The model under review builds one solid part; all positions refer to its coordinate system, in mm. A direction names the side the tool comes from. Coordinates: 2 decimals unless noted, no trailing zeros. Loops run counter-clockwise (first coordinate to the right, second up) from the corner with the lowest first, then second, coordinate; pieces in that order, holes last. Notation, with made-up numbers: M 75,46 L 98,46 A27 ccw 98,72 Z; hole C 46.25,21.25 d1. An arc over 180 degrees is marked long. Use CSV: the item, a comma, the result in double quotes. Start each with the question number.
1. Draft analysis for pull direction X (two halves, no side actions). For faces 5 (the flat face through (-32, 2, -32.258)), 6 (the flat face through (-42.037, 2, 0)), 7 (the flat face through (-1, -5.08, -9)), state which applies: +X half, -X half, draft (parallel to the pull), parting line (faces both ways), or undercut.
2. Add section B-B, the plane z = 0. Write out the cut boundary in (x, y).
3. Clearance check with flat-ended pins moving along their axes: P1, Ø8, axis at x = -18.5, z = 4.5, coming from the +Y side; P2, Ø4, axis at x = -28.5, z = 27, coming from the -Y side; P3, Ø5.5, axis at y = 2.5, z = -32, coming from the +X side; P4, Ø2.5, axis at y = 5.5, z = 34, coming from the +X side. State where each tip first meets the part, or that it passes through.
4. For L1, parallel to Z at x = -15, y = -2.25; L2, parallel to Z at x = 6, y = 9.25; L3, parallel to Z at x = 28, y = 9, list the stretches that pass through material, from the lowest coordinate up.
5. Add section C-C, the plane x = 0. Write out the cut boundary in (y, z), then the cut area to 3 significant figures.
6. Add section A-A, the plane x = -10. Write out the cut boundary in (y, z).
7. Tool access review of faces 1 (the flat face through (0, 2, -38.862)), 2 (the flat face through (1, 5.08, 7)), 3 (the flat face through (37.973, 2, -27)), 4 (the flat face through (1, 8, 22.733)): name each direction out of +Z, -Z, +X, -X, +Y, -Y from which nothing blocks a thin tool from reaching the whole face with its end or side.
8. Add section D-D, the plane y = -0.75. State how many separate pieces and enclosed holes the cut face has, then the cut area to 3 significant figures.
from build123d import *

# Parameters (mm, degrees)
SKETCH1_W                = 84.074
SKETCH1_H                = 77.724
BOSS_EXTRUDE1_DEPTH      = 5.08
BOSS_EXTRUDE1_DEPTH_BACK = 5.08
SKETCH2_W                = 84.074
SKETCH2_H                = 77.724
BOSS_EXTRUDE2_DEPTH      = 5.08
BOSS_EXTRUDE2_DEPTH_BACK = 10.16
SKETCH3_W                = 53.086
SKETCH3_H                = 5.08
CUT_EXTRUDE1_DEPTH       = 6.08
CUT_EXTRUDE1_DEPTH_BACK  = 11.16
SKETCH4_W                = 75.946
SKETCH4_H                = 5.08
CUT_EXTRUDE2_DEPTH       = 6.08
CUT_EXTRUDE2_DEPTH_BACK  = 11.16
SKETCH5_W                = 75.946
SKETCH5_H                = 7.62
BOSS_EXTRUDE3_DEPTH      = 5.08
BOSS_EXTRUDE3_DEPTH_BACK = 10.16
SKETCH10_R               = 5.08
CUT_EXTRUDE4_DEPTH       = 6.08
CUT_EXTRUDE4_DEPTH_BACK  = 11.16
FILLET1_R                = 10.16
CUT_EXTRUDE6_START       = -16.24
SKETCH15_R               = 2.54
SKETCH15_W               = 7.62
SKETCH15_H               = 3.048
CUT_EXTRUDE6_DEPTH       = 17.24
SKETCH7_W                = 34.036
SKETCH7_H                = 5.08
CUT_EXTRUDE7_DEPTH       = 5.064
SKETCH14_W               = 64.77
SKETCH14_H               = 3.81
SKETCH14_W_2             = 63.5
SKETCH14_H_2             = 3.429
CUT_EXTRUDE8_DEPTH       = 3.81


with BuildPart() as part:
    # Sketch1 → Boss-Extrude1 (new body, two sides)
    with BuildSketch(Plane(origin=(0, 0, 0), x_dir=(1, 0, 0), z_dir=(0, 1, 0))) as boss_extrude1_sk:
        Rectangle(SKETCH1_W, SKETCH1_H)
    extrude(amount=BOSS_EXTRUDE1_DEPTH)
    extrude(boss_extrude1_sk.sketch, amount=-BOSS_EXTRUDE1_DEPTH_BACK)

    # Sketch2 → Boss-Extrude2 (add, two sides)
    with BuildSketch(Plane(origin=(0, 5.08, 0), x_dir=(1, 0, 0), z_dir=(0, 1, 0))) as boss_extrude2_sk:
        Rectangle(SKETCH2_W, SKETCH2_H)
        Polygon((-37.973, -29.718), (-37.973, 29.718), (-25.273, 29.718), (-25.273, 34.798), (27.813, 34.798), (27.813, 29.718), (37.973, 29.718), (37.973, -29.718), (27.813, -29.718), (27.813, -34.798), (-25.273, -34.798), (-25.273, -29.718), align=None, mode=Mode.SUBTRACT)
    extrude(amount=BOSS_EXTRUDE2_DEPTH)
    extrude(boss_extrude2_sk.sketch, amount=-BOSS_EXTRUDE2_DEPTH_BACK)

    # Sketch3 → Cut-Extrude1 (cut, two sides)
    with BuildSketch(Plane(origin=(0, 5.08, 0), x_dir=(1, 0, 0), z_dir=(0, 1, 0))) as cut_extrude1_sk:
        with Locations((1.27, 32.258)):
            Rectangle(SKETCH3_W, SKETCH3_H)
        with Locations((1.27, -32.258)):
            Rectangle(SKETCH3_W, SKETCH3_H)
    extrude(amount=CUT_EXTRUDE1_DEPTH, mode=Mode.SUBTRACT)
    extrude(cut_extrude1_sk.sketch, amount=-CUT_EXTRUDE1_DEPTH_BACK, mode=Mode.SUBTRACT)

    # Sketch4 → Cut-Extrude2 (cut, two sides)
    with BuildSketch(Plane(origin=(0, 5.08, 0), x_dir=(1, 0, 0), z_dir=(0, 1, 0))) as cut_extrude2_sk:
        with Locations((0, 27.178)):
            Rectangle(SKETCH4_W, SKETCH4_H)
        with Locations((0, -27.178)):
            Rectangle(SKETCH4_W, SKETCH4_H)
    extrude(amount=CUT_EXTRUDE2_DEPTH, mode=Mode.SUBTRACT)
    extrude(cut_extrude2_sk.sketch, amount=-CUT_EXTRUDE2_DEPTH_BACK, mode=Mode.SUBTRACT)

    # Sketch5 → Boss-Extrude3 (add, two sides)
    with BuildSketch(Plane(origin=(0, 5.08, 0), x_dir=(1, 0, 0), z_dir=(0, 1, 0))) as boss_extrude3_sk:
        with Locations((0, 20.828)):
            Rectangle(SKETCH5_W, SKETCH5_H)
        with Locations((0, -20.828)):
            Rectangle(SKETCH5_W, SKETCH5_H)
    extrude(amount=BOSS_EXTRUDE3_DEPTH)
    extrude(boss_extrude3_sk.sketch, amount=-BOSS_EXTRUDE3_DEPTH_BACK)

    # Sketch10 → Cut-Extrude4 (cut, two sides)
    with BuildSketch(Plane(origin=(0, 5.08, 0), x_dir=(1, 0, 0), z_dir=(0, 1, 0))) as cut_extrude4_sk:
        with Locations((3.937, 0)):
            Circle(SKETCH10_R)
    extrude(amount=CUT_EXTRUDE4_DEPTH, mode=Mode.SUBTRACT)
    extrude(cut_extrude4_sk.sketch, amount=-CUT_EXTRUDE4_DEPTH_BACK, mode=Mode.SUBTRACT)

    # Fillet1
    fillet1_edges = [part.edges().sort_by_distance(p)[0] for p in [
        (42.037, 2.54, 38.862),
        (-42.037, 2.54, 38.862),
        (-42.037, 2.54, -38.862),
        (42.037, 2.54, -38.862),
    ]]
    fillet(fillet1_edges, radius=FILLET1_R)

    # Sketch15 → Cut-Extrude6 (cut)
    with BuildSketch(Plane(origin=(0, 10.16, 0), x_dir=(1, 0, 0), z_dir=(0, 1, 0)).offset(CUT_EXTRUDE6_START)):
        with Locations((32.893, 34.29)):
            Circle(SKETCH15_R)
        with Locations((-31.877, 33.782)):
            Rectangle(SKETCH15_W, SKETCH15_H)
    cut_extrude6 = extrude(amount=CUT_EXTRUDE6_DEPTH, mode=Mode.SUBTRACT)

    # Mirror1: Cut-Extrude6 across plane
    add(cut_extrude6.mirror(Plane.XY), mode=Mode.SUBTRACT)

    # Sketch7 → Cut-Extrude7 (cut, through all)
    with BuildSketch(Plane.ZY.offset(-37.973)):
        with Locations((0, 7.62)):
            Rectangle(SKETCH7_W, SKETCH7_H)
    extrude(amount=-CUT_EXTRUDE7_DEPTH, mode=Mode.SUBTRACT)

    # Sketch14 → Cut-Extrude8 (cut)
    with BuildSketch(Plane(origin=(0, 10.16, 0), x_dir=(1, 0, 0), z_dir=(0, 1, 0))):
        with Locations((1.015527002, -20.828)):
            Rectangle(SKETCH14_W, SKETCH14_H)
        with Locations((0.914410511, 20.828)):
            Rectangle(SKETCH14_W_2, SKETCH14_H_2)
    extrude(amount=-CUT_EXTRUDE8_DEPTH, mode=Mode.SUBTRACT)


solid = part.part
Computed:
1,face 5,"undercut"
1,face 6,"-X half"
1,face 7,"draft"
2,outline,"M -42.04,-5.08 L -1.14,-5.08 L -1.14,5.08 L -37.97,5.08 L -37.97,10.16 L -42.04,10.16 Z; M 9.02,-5.08 L 42.04,-5.08 L 42.04,5.08 L 9.02,5.08 Z"
3,P1,"stops at y = 5.08"
3,P2,"passes through"
3,P3,"stops at x = 42.02"
3,P4,"stops at x = 41.2"
4,L1,"z = -38.86 to -34.8, -24.64 to 24.64, 34.8 to 38.86"
4,L2,"z = -38.86 to -34.8, -24.64 to -22.54, -19.11 to -17.02, 17.02 to 18.92, 22.73 to 24.64, 34.8 to 38.86"
4,L3,"z = -38.86 to -29.72, -24.64 to -22.54, -19.11 to -17.02, 17.02 to 18.92, 22.73 to 24.64, 29.72 to 38.86"
5,outline,"M -5.08,-38.86 L 10.16,-38.86 L 10.16,-34.8 L -5.08,-34.8 Z; M -5.08,-24.64 L 10.16,-24.64 L 10.16,-22.54 L 6.35,-22.54 L 6.35,-19.11 L 10.16,-19.11 L 10.16,-17.02 L 5.08,-17.02 L 5.08,-3.21 L -5.08,-3.21 Z; M -5.08,3.21 L 5.08,3.21 L 5.08,17.02 L 10.16,17.02 L 10.16,18.92 L 6.35,18.92 L 6.35,22.73 L 10.16,22.73 L 10.16,24.64 L -5.08,24.64 Z; M -5.08,34.8 L 10.16,34.8 L 10.16,38.86 L -5.08,38.86 Z"
5,area,"609 mm^2"
6,outline,"M -5.08,-38.86 L 10.16,-38.86 L 10.16,-34.8 L -5.08,-34.8 Z; M -5.08,-24.64 L 10.16,-24.64 L 10.16,-22.54 L 6.35,-22.54 L 6.35,-19.11 L 10.16,-19.11 L 10.16,-17.02 L 5.08,-17.02 L 5.08,17.02 L 10.16,17.02 L 10.16,18.92 L 6.35,18.92 L 6.35,22.73 L 10.16,22.73 L 10.16,24.64 L -5.08,24.64 Z; M -5.08,34.8 L 10.16,34.8 L 10.16,38.86 L -5.08,38.86 Z"
7,face 1,"-Z, +X, -X, +Y, -Y"
7,face 2,"+X, +Y"
7,face 3,"+Y, -Y"
7,face 4,"+Y"
8,separate pieces,"1"
8,enclosed holes,"7"
8,area,"4,970 mm^2"
